Input: part model. Units: mm. Frame: model coordinates. A direction names the side the tool comes from. Round coordinates to 2 decimals unless told otherwise and drop trailing zeros. Loops run counter-clockwise (first coordinate to the right, second up) from the corner with the lowest first, then second, coordinate; pieces in that order, holes last. Notation, with made-up numbers: (59, 62.25) -> (85, 62.25) arc R7 ccw to (85, 74.25) -> close; hole circle Ø2 at (10.25, 12.25). An arc over 180 degrees is marked (long way). Answer as a JSON object with one key per item and string values.
```python
from build123d import *

# Parameters (mm, degrees)
F1_DEPTH = 76.2
F2_R     = 12.7
F3_DEPTH = 76.201
F5_DEPTH = 25.401
F6_R     = 38.1
F9_DEPTH = 6.35


# Not quite as in the source:
# - a pattern or mirror of a feature is missing from the dataset's text; its kind, count and spacing are read off the source's solid


with BuildPart() as f1:
    # F0 (on Front) → F1 (new body, symmetric)
    with BuildSketch(Plane.XZ):
        Polygon((-76.2, 0), (0, 0), (0, 152.4), (-25.4, 152.4), (-25.4, 25.4), (-76.2, 25.4), align=None)
    extrude(amount=F1_DEPTH, both=True)

    # F2 (on Right) → F3 (cut, through all)
    with BuildSketch(Plane.YZ):
        with Locations((0, 114.3)):
            Circle(F2_R)
    extrude(amount=-F3_DEPTH, mode=Mode.SUBTRACT)

    # F4 (on face) → F5 (cut, through all)
    with BuildSketch(Plane.XY.offset(25.4)):
        with BuildLine():
            Line((-63.5, 25.4), (-76.2, 25.4))
            Line((-76.2, 25.4), (-76.2, -25.4))
            Line((-76.2, -25.4), (-63.5, -25.4))
            ThreePointArc((-63.5, -25.4), (-38.1, 0), (-63.5, 25.4))
        make_face()
    extrude(amount=-F5_DEPTH, mode=Mode.SUBTRACT)

    # F6
    f6_edges = [f1.edges().sort_by_distance(p)[0] for p in [
        (-12.7, -76.2, 152.4),
        (-12.7, 76.2, 152.4),
    ]]
    fillet(f6_edges, radius=F6_R)

    # F8 (on offset) → F9 (join, symmetric)
    with BuildSketch(Plane.XZ.offset(44.45)):
        Polygon((-50.8, 25.4), (-25.4, 25.4), (-25.4, 101.6), align=None)
    f9 = extrude(amount=F9_DEPTH, both=True)

    # F9_copies: F9 across plane
    add(f9.mirror(Plane.ZX))


solid = f1.part
```
1) Ray query, probe 1 along Z at (x, y) = (-15.5, 0); probe 2 along Y at (x, z) = (-7, 114); probe 3 along Y at (x, z) = (-33, 77.5). Return the intervals inside material, ascending.
Output:
{"probe 1": "z = 0 to 101.6, 127 to 152.4", "probe 2": "y = -76.2 to -12.7, 12.7 to 76.2", "probe 3": "y = -50.8 to -38.1, 38.1 to 50.8"}
2) Reachability of faces 5 (the face through (-25.4, -1, 90)), 6 (the face through (-33, 50.8, 47)), 7 (the face through (-33, -50.8, 47)), 8 (the face through (-22, 76.2, 45)), 9 (the face through (-70, -25.4, 13)) from +Z, -Z, +X, -X, +Y, -Y: full face, straight path, thin tool, end or side. Return the list, or none.
Output:
{"face 5": "+Z, -X", "face 6": "+Z, -X, +Y", "face 7": "+Z, -X, -Y", "face 8": "+Z, -Z, +X, -X, +Y", "face 9": "+Z, -Z, -X"}
3) Draft query along Y for faces 1 (the face through (-30, -1, 0)), 2 (the face through (-33, -38.1, 47)), 3 (the face through (-70, 25.4, 13)), 4 (the face through (-12.88, -65.34, 140.94)). Return one class per face: +Y half, -Y half, draft (parallel to the pull), parting line (faces both ways), or undercut.
Output:
{"face 1": "draft", "face 2": "undercut", "face 3": "undercut", "face 4": "-Y half"}
4) Section D-D, the plane z = 17. Output: boundary loops of the cut face in (x, y), plus the area to 3 significant figures.
Output:
{"outline": "(-76.2, -76.2) -> (0, -76.2) -> (0, 76.2) -> (-76.2, 76.2) -> (-76.2, 25.4) -> (-63.5, 25.4) arc R25.4 cw to (-63.5, -25.4) -> (-76.2, -25.4) -> close", "area": "9,950 mm^2"}
5) Contact query for flat-ended pins moving along their axis: P1, Ø12.5, axis at x = -44.5, z = 54.5, coming from the -Y side; P2, Ø15, axis at x = -47, y = -23.5, coming from the +Z side; P3, Ø10, axis at y = 48, z = 52.5, coming from the -X side. Output: stop coordinate, or through.
Output:
{"P1": "stops at y = -50.8", "P2": "stops at z = 25.4", "P3": "stops at x = -43.43"}
6) Section B-B, the plane y = 0. Output: boundary loops of the cut face in (x, z), plus the area to 3 significant figures.
Output:
{"outline": "(-38.1, 0) -> (0, 0) -> (0, 101.6) -> (-25.4, 101.6) -> (-25.4, 25.4) -> (-38.1, 25.4) -> close; (-25.4, 127) -> (0, 127) -> (0, 152.4) -> (-25.4, 152.4) -> close", "area": "3,550 mm^2"}
7) Section A-A, the plane x = -71. Output: boundary loops of the cut face in (y, z), plus the area to 3 significant figures.
Output:
{"outline": "(-76.2, 0) -> (-25.4, 0) -> (-25.4, 25.4) -> (-76.2, 25.4) -> close; (25.4, 0) -> (76.2, 0) -> (76.2, 25.4) -> (25.4, 25.4) -> close", "area": "2,580 mm^2"}
8) Section C-C, the plane x = -13. Output: boundary loops of the cut face in (y, z).
Output:
{"outline": "(-76.2, 0) -> (76.2, 0) -> (76.2, 114.3) arc R38.1 ccw to (38.1, 152.4) -> (-38.1, 152.4) arc R38.1 ccw to (-76.2, 114.3) -> close; hole circle Ø25.4 at (0, 114.3)"}
